Geometry: final body of the model. Coordinates: model frame, mm. A direction names the side the tool comes from. Give positions to 0.01 mm unless a question says otherwise; leave off trailing zeros. Write each loop counter-clockwise with the first axis right and the second up, starting at its lowest first coordinate (ties: lowest second). Pieces come first, ordered by that corner, then holes. Notation, with made-up numbers: M -38.5,-25 L -32.5,-25 A24 ccw -32.5,-15 Z; hole C -4,14.5 d4. An arc over 180 degrees is marked long. Use a Markdown table: item, result. Add a question column.
1) Section C-C on y = 0.55. Return the cut outline in (x, z).
2) Draft query along Y for faces 1 (the flat face through (0, 1.15, -4)), 2 (the flat face through (0, 2, 9.8)), 3 (the flat face through (-2.71, 5.1, 11.6)). Return one class per face: +Y half, -Y half, draft (parallel to the pull), parting line (faces both ways), or undercut.
3) Section B-B on y = 3.55. Return the cut outline in (x, z), then the cut area to 3 significant figures.
4) Section D-D on z = 10.5. Return the cut outline in (x, y).
5) Pin query (flat end, axial travel): pin 1 (1 mm diameter, centred on x = -2.5, z = 1, fed in from +Y); pin 2 (0.5 mm diameter, centred on x = -2, y = 2, fed in from +Z); pin 3 (1 mm diameter, centred on x = 8, y = 2, fed in from -Z); pin 4 (0.8 mm diameter, centred on y = 2, z = 8.5, fed in from -X). Return the tip coordinate at first contact, or that it passes through.
6) Set-up query: faces 4 (the flat face through (0, 2.8, 8)), 5 (the flat face through (-0.2, 0.5, 11.8)), 6 (the flat face through (2.21, 5.1, 11.6)). Return all of +Z, -Z, +X, -X, +Y, -Y with unobstructed straight access to the full face (end or side cutting, diameter ignored); none if empty.
7) Section A-A on x = -10.3. Return the cut outline in (y, z), then the cut area to 3 significant figures.
8) Line query: line 1 (X direction, y = 0.7, z = 10.3); line 2 (Y direction, x = 2.25, z = 11.5). Output: solid intervals per line, ascending.
```python
from build123d import *

# Parameters (mm, degrees)
SKETCH_1_W                         = 23.6
SKETCH_1_H                         = 23.6
EXTRUDE_1_DEPTH                    = 1.1
CUT_EXTRUDE_1_REACH                = 18.724
SKETCH_2_R                         = 1.15
MIRROR_2_COPY_1_REACH              = 18.724
MIRROR_2_COPY_1_SKETCH_R           = 1.15
SKETCH_3_W                         = 7.4
SKETCH_3_H                         = 2.4
EXTRUDE_2_DEPTH                    = 1.7
EXTRUDE_3_DEPTH                    = 0.25
CHAMFER_7_SIZE                     = 0.1
FILLET_1_R                         = 0.3
FILLET_2_R                         = 0.8
PATTERN_LINEAR_2_COUNT             = 2
PATTERN_LINEAR_2_PITCH             = 2.46
CHAMFER_7_OF_PATTERN_LINEAR_2_SIZE = 0.1
FILLET_1_OF_PATTERN_LINEAR_2_R     = 0.3
FILLET_2_OF_PATTERN_LINEAR_2_R     = 0.8
PATTERN_LINEAR_3_COUNT             = 2
PATTERN_LINEAR_3_PITCH             = 2.46
CHAMFER_7_OF_PATTERN_LINEAR_3_SIZE = 0.1
FILLET_1_OF_PATTERN_LINEAR_3_R     = 0.3
FILLET_2_OF_PATTERN_LINEAR_3_R     = 0.8
EXTRUDE_START                      = 0.55
SKETCH_7_R                         = 6.4
EXTRUDE_10_DEPTH                   = 0.6
SKETCH_8_W                         = 8.601343457
SKETCH_8_H                         = 2.116418894
CUT_EXTRUDE_2125_DEPTH             = 1.6


with BuildPart() as part:
    # 草图1 → 凸台-拉伸1 (new body)
    with BuildSketch(Plane(origin=(0, 0, 0), x_dir=(1, 0, 0), z_dir=(0, 1, 0))):
        Rectangle(SKETCH_1_W, SKETCH_1_H)
    extrude(amount=EXTRUDE_1_DEPTH)

    # 草图2 → 切除-拉伸1 (cut, up to next)
    with BuildSketch(Plane(origin=(0, 1.1, 0), x_dir=(1, 0, 0), z_dir=(0, 1, 0)), mode=Mode.PRIVATE) as cut_extrude_1_sk1:
        with Locations(Location((10.3, -10.3, 0), (0, 0, 270))):
            Circle(SKETCH_2_R)
    cut_extrude_1_tool1 = extrude(cut_extrude_1_sk1.sketch, amount=-CUT_EXTRUDE_1_REACH, mode=Mode.PRIVATE) & part.part
    cut_extrude_1 = cut_extrude_1_tool1.solids().sort_by_distance((10.3, 1.1, 10.3))[0]
    add(cut_extrude_1, mode=Mode.SUBTRACT)

    # 镜向1: 切除-拉伸1 across plane
    add(cut_extrude_1.mirror(Plane(origin=(0, 0, 0), x_dir=(0, 0, 1), z_dir=(1, 0, 0))), mode=Mode.SUBTRACT)

    # 镜向2: 切除-拉伸1 across plane
    add(cut_extrude_1.mirror(Plane.XY), mode=Mode.SUBTRACT)

    # 镜向2 copy 1 sketch → 镜向2 copy 1 (cut, up to next)
    with BuildSketch(Plane(origin=(0, 1.1, 0), x_dir=(-1, 0, 0), z_dir=(0, 1, 0)), mode=Mode.PRIVATE) as mirror_2_copy_1_sk1:
        with Locations(Location((10.3, -10.3, 0), (0, 0, 270))):
            Circle(MIRROR_2_COPY_1_SKETCH_R)
    mirror_2_copy_1_tool1 = extrude(mirror_2_copy_1_sk1.sketch, amount=-MIRROR_2_COPY_1_REACH, mode=Mode.PRIVATE) & part.part
    add(mirror_2_copy_1_tool1.solids().sort_by_distance((-10.3, 1.1, -10.3))[0], mode=Mode.SUBTRACT)

    # 草图3 → 凸台-拉伸2 (add)
    with BuildSketch(Plane(origin=(0, 1.1, 0), x_dir=(1, 0, 0), z_dir=(0, 1, 0))):
        with Locations((0, -8.6)):
            Rectangle(SKETCH_3_W, SKETCH_3_H)
    extrude(amount=EXTRUDE_2_DEPTH)

    # 草图4 → 凸台-拉伸3 (add, symmetric)
    with BuildSketch(Plane(origin=(0, 0, 0), x_dir=(0, 0, -1), z_dir=(1, 0, 0))):
        Polygon((-8.35, -1.6), (-8.35, 5.4), (-16.15, 5.4), (-16.15, 4.9), (-8.85, 4.9), (-8.85, -1.6), align=None)
    extrude_3 = extrude(amount=EXTRUDE_3_DEPTH, both=True)

    # 倒角7
    chamfer_7_edges = [part.edges().sort_by_distance(p)[0] for p in [
        (0, -1.6, 8.35),
        (0.25, -1.6, 8.6),
        (-0.25, -1.6, 8.6),
        (0, -1.6, 8.85),
        (-0.25, 5.15, 16.15),
        (0, 5.4, 16.15),
        (0, 4.9, 16.15),
        (0.25, 5.15, 16.15),
    ]]
    chamfer(chamfer_7_edges, length=CHAMFER_7_SIZE)

    # 圆角1
    fillet_1_edges = [part.edges().sort_by_distance(p)[0] for p in [
        (0, 4.9, 8.85),
    ]]
    fillet(fillet_1_edges, radius=FILLET_1_R)

    # 圆角2
    fillet_2_edges = [part.edges().sort_by_distance(p)[0] for p in [
        (0, 5.4, 8.35),
    ]]
    fillet(fillet_2_edges, radius=FILLET_2_R)

    # 阵列(线性)2: 凸台-拉伸3 ×2
    with Locations(*[(i * PATTERN_LINEAR_2_PITCH, 0, 0) for i in range(1, PATTERN_LINEAR_2_COUNT)]):
        add(extrude_3)

    # 倒角7 of 阵列(线性)2
    chamfer_7_of_pattern_linear_2_edges = [part.edges().sort_by_distance(p)[0] for p in [
        (2.46, -1.6, 8.35),
        (2.71, -1.6, 8.6),
        (2.21, -1.6, 8.6),
        (2.46, -1.6, 8.85),
        (2.21, 5.15, 16.15),
        (2.46, 5.4, 16.15),
        (2.46, 4.9, 16.15),
        (2.71, 5.15, 16.15),
    ]]
    chamfer(chamfer_7_of_pattern_linear_2_edges, length=CHAMFER_7_OF_PATTERN_LINEAR_2_SIZE)

    # 圆角1 of 阵列(线性)2
    fillet_1_of_pattern_linear_2_edges = [part.edges().sort_by_distance(p)[0] for p in [
        (2.46, 4.9, 8.85),
    ]]
    fillet(fillet_1_of_pattern_linear_2_edges, radius=FILLET_1_OF_PATTERN_LINEAR_2_R)

    # 圆角2 of 阵列(线性)2
    fillet_2_of_pattern_linear_2_edges = [part.edges().sort_by_distance(p)[0] for p in [
        (2.46, 5.4, 8.35),
    ]]
    fillet(fillet_2_of_pattern_linear_2_edges, radius=FILLET_2_OF_PATTERN_LINEAR_2_R)

    # 阵列(线性)3: 凸台-拉伸3 ×2
    with Locations(*[(-i * PATTERN_LINEAR_3_PITCH, 0, 0) for i in range(1, PATTERN_LINEAR_3_COUNT)]):
        add(extrude_3)

    # 倒角7 of 阵列(线性)3
    chamfer_7_of_pattern_linear_3_edges = [part.edges().sort_by_distance(p)[0] for p in [
        (-2.46, -1.6, 8.35),
        (-2.21, -1.6, 8.6),
        (-2.71, -1.6, 8.6),
        (-2.46, -1.6, 8.85),
        (-2.71, 5.15, 16.15),
        (-2.46, 5.4, 16.15),
        (-2.46, 4.9, 16.15),
        (-2.21, 5.15, 16.15),
    ]]
    chamfer(chamfer_7_of_pattern_linear_3_edges, length=CHAMFER_7_OF_PATTERN_LINEAR_3_SIZE)

    # 圆角1 of 阵列(线性)3
    fillet_1_of_pattern_linear_3_edges = [part.edges().sort_by_distance(p)[0] for p in [
        (-2.46, 4.9, 8.85),
    ]]
    fillet(fillet_1_of_pattern_linear_3_edges, radius=FILLET_1_OF_PATTERN_LINEAR_3_R)

    # 圆角2 of 阵列(线性)3
    fillet_2_of_pattern_linear_3_edges = [part.edges().sort_by_distance(p)[0] for p in [
        (-2.46, 5.4, 8.35),
    ]]
    fillet(fillet_2_of_pattern_linear_3_edges, radius=FILLET_2_OF_PATTERN_LINEAR_3_R)

    # 草图7 → 凸台-拉伸10 (add, symmetric)
    with BuildSketch(Plane(origin=(0, 0, 0), x_dir=(1, 0, 0), z_dir=(0, 1, 0)).offset(EXTRUDE_START)):
        with Locations(Location((0, 4.4, 0), (0, 0, 270))):
            Circle(SKETCH_7_R)
    extrude(amount=EXTRUDE_10_DEPTH, both=True)

    # 草图8 → Cut-Extrude 2125 (cut)
    with BuildSketch(Plane.XZ):
        with Locations((-0.203501817, 8.619224199)):
            Rectangle(SKETCH_8_W, SKETCH_8_H)
    extrude(amount=CUT_EXTRUDE_2125_DEPTH, mode=Mode.SUBTRACT)


solid = part.part
```
Found:
| question | item | result |
|---|---|---|
| 1 | outline | M -11.8,-11.8 L 11.8,-11.8 L 11.8,11.8 L -11.8,11.8 Z; hole C -10.3,-10.3 d2.3; hole C -10.3,10.3 d2.3; hole C 10.3,-10.3 d2.3; hole C 10.3,10.3 d2.3 |
| 2 | face 1 | +Y half |
| 2 | face 2 | undercut |
| 2 | face 3 | draft |
| 3 | outline | M -2.71,8.35 L -2.21,8.35 L -2.21,8.85 L -2.71,8.85 Z; M -0.25,8.35 L 0.25,8.35 L 0.25,8.85 L -0.25,8.85 Z; M 2.21,8.35 L 2.71,8.35 L 2.71,8.85 L 2.21,8.85 Z |
| 3 | area | 0.750 mm² |
| 4 | outline | M -11.8,0 L -11.43,0 L -11.43,1.1 L -11.8,1.1 Z; M -9.17,0 L 9.17,0 L 9.17,1.1 L -9.17,1.1 Z; M -2.71,4.9 L -2.21,4.9 L -2.21,5.4 L -2.71,5.4 Z; M -0.25,4.9 L 0.25,4.9 L 0.25,5.4 L -0.25,5.4 Z; M 2.21,4.9 L 2.71,4.9 L 2.71,5.4 L 2.21,5.4 Z; M 11.43,0 L 11.8,0 L 11.8,1.1 L 11.43,1.1 Z |
| 5 | pin 1 | y = 1.15 |
| 5 | pin 2 | z = 9.8 |
| 5 | pin 3 | through |
| 5 | pin 4 | x = -3.7 |
| 6 | face 4 | none |
| 6 | face 5 | +Z, +X, -X, -Y |
| 6 | face 6 | +Z, -Z, +Y |
| 7 | outline | M 0,-11.8 L 1.1,-11.8 L 1.1,-11.45 L 0,-11.45 Z; M 0,-9.15 L 1.1,-9.15 L 1.1,9.15 L 0,9.15 Z; M 0,11.45 L 1.1,11.45 L 1.1,11.8 L 0,11.8 Z |
| 7 | area | 20.9 mm² |
| 8 | line 1 | -11.8 to -11.45, -9.15 to 9.15, 11.45 to 11.8 |
| 8 | line 2 | 0 to 1.1, 4.9 to 5.4 |
